Job drawing, mm, ordinate dimensions from the low corner. One solid piece. A direction names the side the tool comes from. Round coordinates to 2 decimals unless told otherwise and drop trailing zeros. Loops run counter-clockwise (first coordinate to the right, second up) from the corner with the lowest first, then second, coordinate; pieces in that order, holes last. Notation, with made-up numbers: M 51.5,80.5 L 71.5,80.5 A32 cw 71.5,106.5 Z; hole C -11.5,18 d10. An arc over 180 degrees is marked long. Use a Markdown table: item, result. Add a question column.
(1) Band-saw the part on D-D, the plane y = 110.5. Write the cut outline in (x, z), and give its area (3 significant figures).
(2) Band-saw the part on A-A, the plane x = 288.5. Write the cut outline in (y, z) (1 decimal), and give its area (3 significant figures).
(3) Flat gauge pins, fed straight in: P1, Ø3, axis at x = 138, z = 354, coming from the +Y side; P2, Ø4, axis at y = 137, z = 227, coming from the -X side; P3, Ø3, axis at x = 317, y = 298.5, coming from the +Z side. Where does each tip first touch, or does it go through?
(4) Band-saw the part on C-C, the plane x = 377.5. Write the cut outline in (y, z).
(5) Band-saw the part on B-B, the plane z = 246.5. Write the cut outline in (x, y) (1 decimal), and give its area (3 significant figures).
(6) Which spindle directions (+Z, -Z, +X, -X, +Y, -Y) get a long thin tool onto all of the face, cutting with end or side? Do the marked faces 3 and 4. Say none if no direction does.
(7) Wall check: L1, parallel to Z at x = 270, y = 193; L2, parallel to Y at x = 473, z = 356; L3, parallel to Z at x = 372, y = 189.5 (1 decimal). Give the ranges that are in metal, low to high.
(8) Two-plate mould, pull along Z, no slides. Class the marked faces 1 and 2: released by +Z, released by -Z, zero draft, split by the parting line, or undercut.
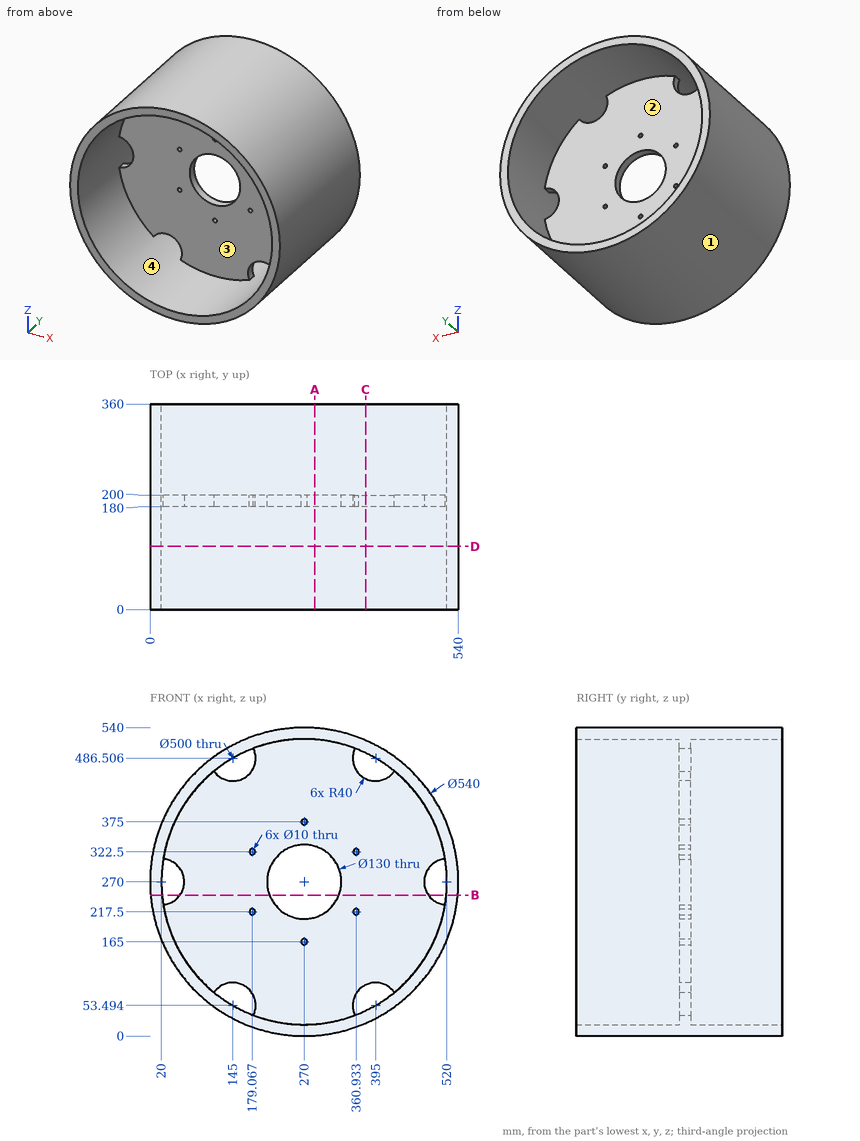
Return value:
| question | item | result |
|---|---|---|
| 1 | outline | C 270,270 d540; hole C 270,270 d500 |
| 1 | area | 32,700 mm^2 |
| 2 | outline | M 0,0.6 L 360,0.6 L 360,20.7 L 200,20.7 L 200,207.7 L 180,207.7 L 180,20.7 L 0,20.7 Z; M 0,519.3 L 180,519.3 L 180,332.3 L 200,332.3 L 200,519.3 L 360,519.3 L 360,539.4 L 0,539.4 Z |
| 2 | area | 21,900 mm^2 |
| 3 | P1 | y = 200 |
| 3 | P2 | x = 3.13 |
| 3 | P3 | z = 536.14 |
| 4 | outline | M 0,22.32 L 360,22.32 L 360,44.29 L 0,44.29 Z; M 0,495.71 L 360,495.71 L 360,517.68 L 0,517.68 Z; M 180,89.46 L 200,89.46 L 200,450.54 L 180,450.54 Z |
| 5 | outline | M 1,0 L 21.1,0 L 21.1,360 L 1,360 Z; M 52.4,180 L 209.4,180 L 209.4,200 L 52.4,200 Z; M 330.6,180 L 487.6,180 L 487.6,200 L 330.6,200 Z; M 518.9,0 L 539,0 L 539,360 L 518.9,360 Z |
| 5 | area | 20,700 mm^2 |
| 6 | face 3 | -Y |
| 6 | face 4 | none |
| 7 | L1 | 0 to 160, 170 to 205, 335 to 370, 380 to 540 |
| 7 | L2 | 180 to 200 |
| 7 | L3 | 20 to 41.8, 86.2 to 453.8, 498.2 to 520 |
| 8 | face 1 | split by the parting line |
| 8 | face 2 | undercut |
